Here's the drawing with two shaded views (mm, measured from the low corner). I have some questions. A direction names the side the tool comes from. Give positions to 0.01 mm unless a question says otherwise; leave off trailing zeros. Write each loop counter-clockwise with the first axis right and the second up, starting at its lowest first coordinate (ties: lowest second). Pieces come first, ordered by that corner, then holes. Notation, with made-up numbers: (81.5, -24.75) - (123.5, -24.75) arc R17 ccw to (123.5, -19.75) - close; hole circle Ø2 at (43, 20). An arc over 180 degrees is marked (long way). Use one line per item in the form item = value.
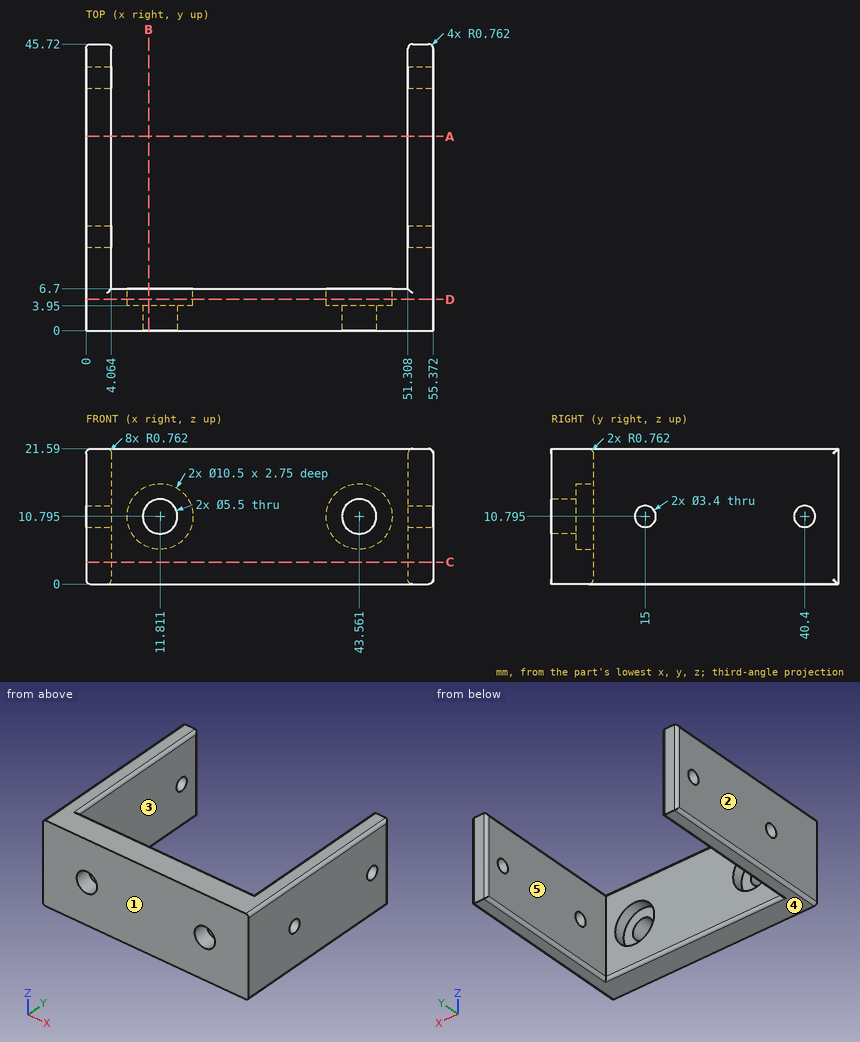
1. Imagine slicing it at B-B, the plane x = 10. List the corners of the cut face in (y, z) for me, and give its area (3 significant figures).
Response values:
outline = (0, 0) - (5.94, 0) arc R0.76 ccw to (6.7, 0.76) - (6.7, 5.87) - (3.95, 5.87) - (3.95, 8.73) - (0, 8.73) - close; (0, 12.86) - (3.95, 12.86) - (3.95, 15.72) - (6.7, 15.72) - (6.7, 20.83) arc R0.76 ccw to (5.94, 21.59) - (0, 21.59) - close
area = 101 mm²
2. Imagine slicing it at C-C, the plane z = 3.5. List the corners of the cut face in (x, y) for me, and give its area (3 significant figures).
Response values:
outline = (0, 0) - (55.37, 0) - (55.37, 44.96) arc R0.76 ccw to (54.61, 45.72) - (52.07, 45.72) arc R0.76 ccw to (51.31, 44.96) - (51.31, 6.7) - (4.06, 6.7) - (4.06, 44.96) arc R0.76 ccw to (3.3, 45.72) - (0.76, 45.72) arc R0.76 ccw to (0, 44.96) - close
area = 688 mm²
3. If we mould it in two halves opening along X, with no side actions, what happens to the marked faces 1, 2 and 3? For each: pulls with the +X half, pulls with the -X half, needs draft (parallel to the pull), parting line crosses it, or undercut.
Response values:
face_1 = needs draft
face_2 = pulls with the -X half
face_3 = undercut
4. Which directions (+Z, -Z, +X, -X, +Y, -Y) give clear straight access to the entire face, cutting with the end or side of a thin tool? Please do the marked faces 4 and 5.
Response values:
face_4 = -Z, +X, -X, +Y, -Y
face_5 = +Z, -Z, +Y
5. For pin 1 (2.5 mm diameter, centred on y = 40.4, z = 10.79, fed in from -X); pin 2 (10 mm diameter, centred on x = 26, z = 12.5, fed in from +Y); pin 3 (5 mm diameter, centred on x = 41.5, z = 12.5, fed in from +Y), each with a flat end and sliding along its axis, tell me the tip position at first contact or that it passes through.
Response values:
pin_1 = through
pin_2 = 6.7
pin_3 = 3.95
6. Imagine slicing it at D-D, the plane y = 5. List the corners of the cut face in (x, z) for me (3 decimals).
Response values:
outline = (0, 0.762) arc R0.762 ccw to (0.762, 0) - (54.61, 0) arc R0.762 ccw to (55.372, 0.762) - (55.372, 20.828) arc R0.762 ccw to (54.61, 21.59) - (0.762, 21.59) arc R0.762 ccw to (0, 20.828) - close; hole circle Ø10.5 at (11.811, 10.795); hole circle Ø10.5 at (43.561, 10.795)
7. Imagine slicing it at A-A, the plane y = 31. List the corners of the cut face in (x, z) for me.
Response values:
outline = (0, 0.76) arc R0.76 ccw to (0.76, 0) - (3.3, 0) arc R0.76 ccw to (4.06, 0.76) - (4.06, 20.83) arc R0.76 ccw to (3.3, 21.59) - (0.76, 21.59) arc R0.76 ccw to (0, 20.83) - close; (51.31, 0.76) arc R0.76 ccw to (52.07, 0) - (54.61, 0) arc R0.76 ccw to (55.37, 0.76) - (55.37, 20.83) arc R0.76 ccw to (54.61, 21.59) - (52.07, 21.59) arc R0.76 ccw to (51.31, 20.83) - close
8. If I drill on line 1 (X direction, y = 25.5, z = 7.75); line 2 (X direction, y = 3, z = 10); line 3 (X direction, y = 4.5, z = 14.25), over which ranges is the centre line in solid material (lowest first)? Write a range as from..to.
Response values:
line_1 = 0..4.06, 51.31..55.37
line_2 = 0..9.18, 14.44..40.93, 46.19..55.37
line_3 = 0..7.86, 15.76..39.61, 47.51..55.37
